from build123d import *

# Parameters (mm, degrees)
F0_W        = 88.9
F0_H        = 88.9
F1_DEPTH    = 88.9
F2_T1_DEPTH = 152.4
F3_T        = -5.08


# Not quite as in the source:
# - a fillet or chamfer that OpenCascade refuses, or shapes differently, is made with other operations: its cross-section is extruded or revolved along the edge and cut away or added


with BuildPart() as f1:
    # F0 (on Top) → F1 (new body)
    with BuildSketch(Plane.XY):
        Rectangle(F0_W, F0_H)
    extrude(amount=F1_DEPTH)

    # F2: fillet of radius 12.7 on 4 edges, made by hand

    # F2_s2 → F2_t1 (cut)
    with BuildSketch(Plane.XY.offset(-31.75)):
        with BuildLine():
            add(Edge.make_bspline(
                [(31.75, -44.45), (44.45, -44.45), (44.45, -31.75)],
                knots=[0, 0, 0, 1, 1, 1], degree=2, weights=[1, 1, 1]))
            Line((44.45, -31.75), (44.45, -44.45))
            Line((44.45, -44.45), (31.75, -44.45))
        make_face()
        with BuildLine():
            add(Edge.make_bspline(
                [(44.45, 31.75), (44.45, 44.45), (31.75, 44.45)],
                knots=[0, 0, 0, 1, 1, 1], degree=2, weights=[1, 1, 1]))
            Line((31.75, 44.45), (44.45, 44.45))
            Line((44.45, 44.45), (44.45, 31.75))
        make_face()
        with BuildLine():
            add(Edge.make_bspline(
                [(-31.75, -44.45), (-44.45, -44.45), (-44.45, -31.75)],
                knots=[0, 0, 0, 1, 1, 1], degree=2, weights=[1, 1, 1]))
            Line((-44.45, -31.75), (-44.45, -44.45))
            Line((-44.45, -44.45), (-31.75, -44.45))
        make_face()
        with BuildLine():
            add(Edge.make_bspline(
                [(-31.75, 44.45), (-44.45, 44.45), (-44.45, 31.75)],
                knots=[0, 0, 0, 1, 1, 1], degree=2, weights=[1, 1, 1]))
            Line((-44.45, 31.75), (-44.45, 44.45))
            Line((-44.45, 44.45), (-31.75, 44.45))
        make_face()
    extrude(amount=F2_T1_DEPTH, mode=Mode.SUBTRACT)

    # F3
    f3_openings = [f1.faces().sort_by_distance(p)[0] for p in [
        (0, 0, 88.9),
    ]]
    offset(amount=F3_T, openings=f3_openings, kind=Kind.INTERSECTION)


solid = f1.part
The model under review builds one solid part; all positions refer to its coordinate system, in mm. A direction names the side the tool comes from. Round coordinates to 2 decimals unless told otherwise and drop trailing zeros. Write each loop counter-clockwise with the first axis right and the second up, starting at its lowest first coordinate (ties: lowest second). Pieces come first, ordered by that corner, then holes. Notation, with made-up numbers: M 73,27 L 104,27 A9 cw 104,41 Z; hole C 62,30 d11. An arc over 180 degrees is marked long. Use a Markdown table: item, result. Add a question column.
Q1. We need section A-A, the plane y = -5. State the section outline as (x, z) points, plus the area to 3 significant figures.
Q2. To check wall thickness, follow line 1 (X direction, y = 1, z = 10.5); line 2 (Z direction, x = -2.5, y = 30). State the ranges of each line that lie inside material, in increasing order.
Q3. Insertion check: pin 1 (12 mm diameter, centred on x = -14, y = 0.5, fed in from +Z). The pin has a flat end and moves straight along its axis. Give the tip position at first contact, or say it passes through.
Q4. Machinability: for faces 1 (the face through (-1, 1, 5.08)), 2 (the face through (0, -44.45, 44)), which of the approach directions +Z, -Z, +X, -X, +Y, -Y give a long, thin tool a straight path to every point of the face, cutting with its end or side? Answer none if there is none.
Q5. The part is to be moulded in two halves that separate along X. For faces 3 (the face through (0, 44.45, 44)), 4 (the face through (-44.45, 0, 44)), 5 (the face through (44.45, 0, 44)), 6 (the face through (39.37, 0, 46)), say which applies: pulls with the +X half, pulls with the -X half, needs draft (parallel to the pull), parting line crosses it, or undercut.
Findings below:
| question | item | result |
|---|---|---|
| 1 | outline | M -44.45,0 L 44.45,0 L 44.45,88.9 L 39.37,88.9 L 39.37,5.08 L -39.37,5.08 L -39.37,88.9 L -44.45,88.9 Z |
| 1 | area | 1,300 mm² |
| 2 | line 1 | x = -44.45 to -39.37, 39.37 to 44.45 |
| 2 | line 2 | z = 0 to 5.08 |
| 3 | pin 1 | stops at z = 5.08 |
| 4 | face 1 | +Z |
| 4 | face 2 | +Z, -Z, +X, -X, -Y |
| 5 | face 3 | needs draft |
| 5 | face 4 | pulls with the -X half |
| 5 | face 5 | pulls with the +X half |
| 5 | face 6 | undercut |
